Geometry: final body of the model. Coordinates: model frame, mm. A direction names the side the tool comes from. Give positions to 0.01 mm unless a question says otherwise; leave off trailing zeros. Write each loop counter-clockwise with the first axis right and the second up, starting at its lowest first coordinate (ties: lowest second). Pieces come first, ordered by that corner, then holes.
Q1. Draft query along Z for faces 1 (the face through (-11.071, -9.808, 2.022)), 2 (the face through (-11, 0, 7.15)), 3 (the face through (8, 0, 0)), 4 (the face through (8.584, 5.46, 4.732)). Return one class per face: pulls with the +Z half, pulls with the -Z half, needs draft (parallel to the pull), parting line crosses it, or undercut.
Q2. Pin query (flat end, axial travel): pin 1 (2.5 mm diameter, centred on x = -2.5, z = 2, fed in from -Y); pin 2 (3 mm diameter, centred on x = -7, y = -3.5, fed in from +Z); pin 3 (9 mm diameter, centred on x = 5.5, y = -3, fed in from +Z). Return the tip coordinate at first contact, or that it passes through.
Q3. Cut plane A-A on y = -5.35. Return the cut outline in (x, z), plus the area to 3 significant figures.
Q4. Cut plane D-D on x = -6. Return the cut outline in (y, z), plus the area to 3 significant figures.
Q5. Cut plane C-C on y = 10.25. Return the cut outline in (x, z).
Q6. Cut plane B-B on z = 4.5. Return the cut outline in (x, y).
Q7. Line query: L1, parallel to Z at x = -11.5, y = -9 (3 decimals); L2, parallel to Y at x = 9.5, z = 5.75; L3, parallel to X at y = 8.75, z = 1.75. Output: solid intervals per line, ascending.
Q8. Reachability of faces 5 (the face through (9, -6, 6)), 6 (the face through (-8.817, 0.091, 3.57)), 7 (the face through (-3, -6.5, 1)), 8 (the face through (3.38, 8.71, 1.48)) from +Z, -Z, +X, -X, +Y, -Y: full face, straight path, thin tool, end or side. Return the list, or none.
```python
from build123d import *

# Parameters (mm, degrees)
PAD006_DEPTH    = 7.15
SKETCH012_W     = 38
SKETCH012_H     = 18
POCKET004_DEPTH = 4.15
SKETCH013_R     = 2.5
PAD007_DEPTH    = 3
SKETCH014_R     = 1.5
POCKET005_DEPTH = 6.001
SKETCH016_W     = 12.5
SKETCH016_H     = 2.5
POCKET006_DEPTH = 5
SKETCH017_R     = 1.75
POCKET007_DEPTH = 5
CHAMFER_SIZE    = 0.5
CHAMFER001_SIZE = 0.5
POCKET008_DEPTH = 25.001
FILLET_R        = 2
FILLET001_R     = 1
FILLET002_R     = 1


with BuildPart() as part:
    # Sketch011 (on XY_Plane001 of Origin002) → Pad006 (new body)
    with BuildSketch(Plane.XY):
        Polygon((-9.418493, -9), (28.581507, -9), (28.581507, 9), (-9.418493, 9), (-9.418493, 12.5), (-12.718493, 12.5), (-12.718493, -12.5), (-9.418493, -12.5), align=None)
    extrude(amount=PAD006_DEPTH)

    # Sketch012 (on Face10 of Pad006) → Pocket004 (cut)
    with BuildSketch(Plane.XY.offset(7.15)):
        with Locations((9.581507, 0)):
            Rectangle(SKETCH012_W, SKETCH012_H)
    extrude(amount=-POCKET004_DEPTH, mode=Mode.SUBTRACT)

    # Sketch013 (on Face4 of Pocket004) → Pad007 (join)
    with BuildSketch(Plane.XY.offset(3)):
        with Locations((11.081507, 5.35)):
            Circle(SKETCH013_R)
        with Locations((11.081507, -5.35)):
            Circle(SKETCH013_R)
    extrude(amount=PAD007_DEPTH)

    # Sketch014 (on Face13 of Pad007) → Pocket005 (cut, through all)
    with BuildSketch(Plane.XY.offset(6)):
        with Locations((11.081507, 5.35)):
            Circle(SKETCH014_R)
        with Locations((11.081507, -5.35)):
            Circle(SKETCH014_R)
    extrude(amount=-POCKET005_DEPTH, mode=Mode.SUBTRACT)

    # Sketch016 (on Face4 of Pocket005) → Pocket006 (cut)
    with BuildSketch(Plane.XY.offset(3)):
        with Locations((-3.168493, 7.75)):
            Rectangle(SKETCH016_W, SKETCH016_H)
        with Locations((-3.168493, -7.75)):
            Rectangle(SKETCH016_W, SKETCH016_H)
    extrude(amount=-POCKET006_DEPTH, mode=Mode.SUBTRACT)

    # Sketch017 (on Face7 of Pocket006) → Pocket007 (cut)
    with BuildSketch(Plane(origin=(-12.718493, 0, 0), x_dir=(0, -1, 0), z_dir=(-1, 0, 0))):
        with Locations((-9, 3.575)):
            Circle(SKETCH017_R)
        with Locations((9, 3.575)):
            Circle(SKETCH017_R)
    extrude(amount=-POCKET007_DEPTH, mode=Mode.SUBTRACT)

    # Chamfer
    chamfer_edges = [part.edges().sort_by_distance(p)[0] for p in [
        (8.581507, 5.35, 3),
        (8.581507, -5.35, 3),
    ]]
    chamfer(chamfer_edges, length=CHAMFER_SIZE)

    # Chamfer001
    chamfer001_edges = [part.edges().sort_by_distance(p)[0] for p in [
        (9.581507, -5.35, 6),
        (9.581507, 5.35, 6),
    ]]
    chamfer(chamfer001_edges, length=CHAMFER001_SIZE)

    # Sketch018 (on Face8 of Chamfer001) → Pocket008 (cut, through all)
    with BuildSketch(Plane.XZ.offset(12.5)):
        Polygon((-12.718493, 7.15), (-12.718493, 0), (-12.518776, 7.15), align=None)
    extrude(amount=-POCKET008_DEPTH, mode=Mode.SUBTRACT)

    # Fillet
    fillet_edges = [part.edges().sort_by_distance(p)[0] for p in [
        (-9.418493, 0, 3),
    ]]
    fillet(fillet_edges, radius=FILLET_R)

    # Fillet001
    fillet001_edges = [part.edges().sort_by_distance(p)[0] for p in [
        (-10.968635, -12.5, 7.15),
        (-10.968635, 12.5, 7.15),
        (-11.068493, -12.5, 0),
        (-11.068493, 12.5, 0),
    ]]
    fillet(fillet001_edges, radius=FILLET001_R)

    # Fillet002
    fillet002_edges = [part.edges().sort_by_distance(p)[0] for p in [
        (3.081507, -9, 1.5),
        (28.581507, -9, 1.5),
        (28.581507, 9, 1.5),
        (3.081507, 9, 1.5),
    ]]
    fillet(fillet002_edges, radius=FILLET002_R)


solid = part.part
```
Data:
1. face 1: undercut
1. face 2: pulls with the +Z half
1. face 3: pulls with the -Z half
1. face 4: needs draft
2. pin 1: stops at y = -6.5
2. pin 2: stops at z = 3.32
2. pin 3: stops at z = 6
3. outline: (-12.72, 0) - (9.58, 0) - (9.58, 5.5) - (9.08, 6) - (8.58, 6) - (8.58, 3.5) - (8.08, 3) - (-7.42, 3) arc R2 cw to (-9.42, 5) - (-9.42, 7.15) - (-12.52, 7.15) - close; (12.58, 0) - (28.58, 0) - (28.58, 3) - (14.08, 3) - (13.58, 3.5) - (13.58, 6) - (13.08, 6) - (12.58, 5.5) - close
3. area: 135 mm2
4. outline: (-6.5, 0) - (6.5, 0) - (6.5, 3) - (-6.5, 3) - close
4. area: 39.0 mm2
5. outline: (-12.72, 0) - (-9.42, 0) - (-9.42, 2.35) - (-12.65, 2.35) - close; (-12.58, 4.8) - (-9.42, 4.8) - (-9.42, 7.15) - (-12.52, 7.15) - close
6. outline: (-12.59, -12.5) - (-9.42, -12.5) - (-9.42, -10.49) - (-12.59, -10.49) - close; (-12.59, -7.51) - (-9.42, -7.51) - (-9.42, -6.5) - (-9.35, -6.5) - (-9.35, 6.5) - (-9.42, 6.5) - (-9.42, 7.51) - (-12.59, 7.51) - close; (-12.59, 10.49) - (-9.42, 10.49) - (-9.42, 12.5) - (-12.59, 12.5) - close; circle Ø5 at (11.08, -5.35); circle Ø5 at (11.08, 5.35); hole circle Ø3 at (11.08, -5.35); hole circle Ø3 at (11.08, 5.35)
7. L1: z = 0 to 1.825, 5.325 to 7.15
7. L2: y = -7.29 to -6.1, -4.6 to -3.41, 3.41 to 4.6, 6.1 to 7.29
7. L3: x = -12.67 to -9.42, 3.42 to 28.24
8. face 5: +Z, +X, +Y, -Y
8. face 6: +Z, +Y, -Y
8. face 7: +Z, -Z, -Y
8. face 8: +Z, -Z, +Y
